from build123d import *

# Parameters (mm, degrees)
F1_DEPTH  = 300
F2_W      = 20
F2_H      = 40
F3_DEPTH  = 50
F5_W      = 25
F5_H      = 20
F6_DEPTH  = 70
F7_R      = 4
F8_DEPTH  = 120
F10_DEPTH = 8
F11_R     = 20
F12_DEPTH = 10
F14_DEPTH = 8


with BuildPart() as f1:
    # F0 (on Right) → F1 (new body)
    with BuildSketch(Plane.YZ):
        Polygon((0, 222.757817), (-102.5, 222.757817), (-12.5, 0), (0, 0), (12.5, 0), (102.5, 222.757817), align=None)
    extrude(amount=F1_DEPTH)

    # F2 (on face) → F3 (join)
    with BuildSketch(Plane(origin=(0, 0, 0), x_dir=(0, -1, 0), z_dir=(-1, 0, 0))):
        with Locations((0, 50)):
            Rectangle(F2_W, F2_H)
    extrude(amount=F3_DEPTH)

    # F5 (on face) → F6 (join)
    with BuildSketch(Plane(origin=(0, 0, 30), x_dir=(1, 0, 0), z_dir=(0, 0, -1))):
        with Locations((-37.5, 0)):
            Rectangle(F5_W, F5_H)
    extrude(amount=F6_DEPTH)

    # F7 (on face) → F8 (cut)
    with BuildSketch(Plane.XY.offset(70)):
        with Locations((-40, 0)):
            Circle(F7_R)
    extrude(amount=-F8_DEPTH, mode=Mode.SUBTRACT)

    # F9 (on face) → F10 (join)
    with BuildSketch(Plane(origin=(0, 0, -40), x_dir=(1, 0, 0), z_dir=(0, 0, -1))):
        Polygon((-50, 0), (-50, -25.201352), (70, -25.201352), (70, -59.376635), (90, -59.376635), (90, 0), (90, 59.376635), (70, 59.376635), (70, 25.201352), (-50, 25.201352), align=None)
    extrude(amount=F10_DEPTH)

    # F11 (on face) → F12 (join)
    with BuildSketch(Plane.XY.offset(-40)):
        with Locations((79.756841, -49.376635)):
            Circle(F11_R)
        with Locations((79.756841, 49.376635)):
            Circle(F11_R)
    extrude(amount=F12_DEPTH)

    # F13 (on face) → F14 (cut)
    with BuildSketch(Plane(origin=(0, 0, -48), x_dir=(1, 0, 0), z_dir=(0, 0, -1))):
        with BuildLine():
            ThreePointArc((80, -4), (84, 0), (80, 4))
            Line((80, 4), (-40, 4))
            ThreePointArc((-40, 4), (-44, 0), (-40, -4))
            Line((-40, -4), (80, -4))
        make_face()
    extrude(amount=-F14_DEPTH, mode=Mode.SUBTRACT)


solid = f1.part
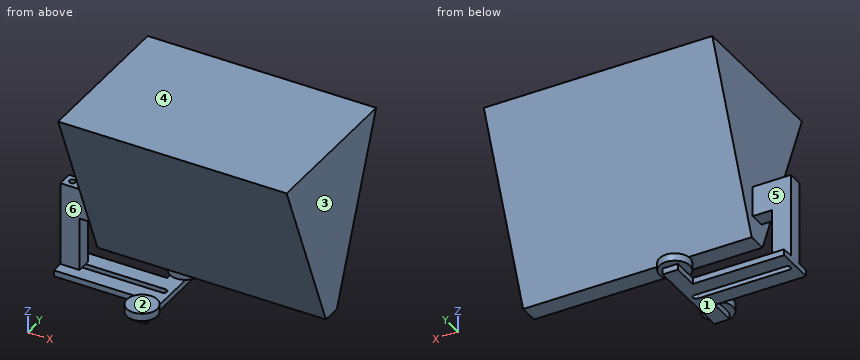
CAD build for the part. Positions are in the model's coordinates, mm. Face numbers are marked on the shaded views. A direction names the side the tool comes from. Round coordinates to 2 decimals unless told otherwise and drop trailing zeros. Write each loop counter-clockwise with the first axis right and the second up, starting at its lowest first coordinate (ties: lowest second). Pieces come first, ordered by that corner, then holes.
(1) Probe line 1 along X through (y, z) = (0, 28); line 2 along Y through (x, z) = (-40, 26.5); line 3 along X through (y, z) = (-19, 94.5). List the from-to ranges inside material, lowest first.
(2) 3-axis set-ups, long thin cutter, end or side, ignore diameter. For the marked faces 4, 5 and 6: which of +Z, -Z, +X, -X, +Y, -Y reach the whole face in a straight line?
(3) Mould opens along Z. For the marked faces 1, 2 and 3 say: pulls with the +Z half, pulls with the -Z half, needs draft (parallel to the pull), parting line crosses it, or undercut.
(4) Slice it at C-C, the plane z = -7.5. Write the cut outline in (x, y).
(5) Slice it at D-D, the plane y = -45. Write the cut outline in (x, z).
(6) Slice it at B-B, the plane y = 0. Write the cut outline in (x, z), and give its area (3 significant figures).
(7) Slice it at A-A, the plane z = 21.5. Write the cut outline in (x, y), and give its area (3 significant figures).
(8) Drop flat-ended pins along their axis: P1, Ø10, axis at x = -36.5, y = 0.5, coming from the +Z side; P2, Ø5, axis at x = 155.5, y = -66, coming from the -Z side; P3, Ø2.5, axis at x = 13.5, z = -45, coming from the +Y side. Give the stop position or say it passes through.
From the geometry:
1. line 1: x = -50 to -44, -36 to -25, 0 to 300
1. line 2: y = -10 to -4, 4 to 10
1. line 3: x = 0 to 300
2. face 4: +Z, +X, -X, +Y, -Y
2. face 5: +Z, -X, +Y
2. face 6: +Z, -X, -Y
3. face 1: pulls with the -Z half
3. face 2: undercut
3. face 3: needs draft
4. outline: (-50, -10) - (-25, -10) - (-25, 10) - (-50, 10) - close; hole circle Ø8 at (-40, 0)
5. outline: (0, 80.44) - (300, 80.44) - (300, 222.76) - (0, 222.76) - close; (60.24, -40) - (70, -40) - (70, -48) - (90, -48) - (90, -40) - (99.27, -40) - (99.27, -30) - (60.24, -30) - close
6. outline: (-50, -48) - (-44, -48) - (-44, 70) - (-50, 70) - close; (-36, -40) - (-25, -40) - (-25, 30) - (0, 30) - (0, 0) - (300, 0) - (300, 222.76) - (0, 222.76) - (0, 70) - (-36, 70) - close; (84, -48) - (90, -48) - (90, -40) - (84, -40) - close
6. area: 69,800 mm2
7. outline: (-50, -10) - (-25, -10) - (-25, 10) - (-50, 10) - close; (0, -21.19) - (300, -21.19) - (300, 21.19) - (0, 21.19) - close; hole circle Ø8 at (-40, 0)
7. area: 13,200 mm2
8. P1: stops at z = 70
8. P2: stops at z = 126.23
8. P3: stops at y = 25.2
